```python
from build123d import *

# Parameters (mm, degrees)
SKETCH1_R           = 10
BOSS_EXTRUDE1_DEPTH = 12
SKETCH2_R           = 2
CUT_EXTRUDE1_DEPTH  = 10
SKETCH3_R           = 0.25
BOSS_EXTRUDE2_DEPTH = 10
SKETCH3_3_R         = 0.25
BOSS_EXTRUDE3_DEPTH = 8


with BuildPart() as part:
    # Sketch1 → Boss-Extrude1 (new body)
    with BuildSketch(Plane.XY):
        Circle(SKETCH1_R)
    extrude(amount=BOSS_EXTRUDE1_DEPTH)

    # Sketch2 → Cut-Extrude1 (cut)
    with BuildSketch(Plane.XY.offset(12)):
        Circle(SKETCH2_R)
    extrude(amount=-CUT_EXTRUDE1_DEPTH, mode=Mode.SUBTRACT)

    # Sketch3 → Boss-Extrude2 (add)
    with BuildSketch(Plane(origin=(0, 0, 0), x_dir=(-1, 0, 0), z_dir=(0, 0, -1))):
        with Locations(Location((-8.5, 0, 0), (0, 0, 180))):
            Circle(SKETCH3_R)
    extrude(amount=BOSS_EXTRUDE2_DEPTH)

    # Sketch3_3 → Boss-Extrude3 (add)
    with BuildSketch(Plane(origin=(0, 0, 0), x_dir=(-1, 0, 0), z_dir=(0, 0, -1))):
        with Locations(Location((8.5, 0, 0), (0, 0, 180))):
            Circle(SKETCH3_3_R)
    extrude(amount=BOSS_EXTRUDE3_DEPTH)


solid = part.part
```
Can you work these out from the model? Positions are in its coordinate system, mm. Coordinates: 2 decimals unless noted, no trailing zeros. Order: outer loops, then holes, each group sorted by start corner. A loop starts at its lowest first (then second) coordinate and runs counter-clockwise, first axis right, second up.
1. If we section it at B-B (z = -5.5): Please give me the cut outline in (x, y).
2. I need wall thicknesses on line 1 (Y direction, x = 0, z = 8); line 2 (Y direction, x = -0.75, z = 4); line 3 (Z direction, x = 5.5, y = 7). Which ranges of each line are inside material? Lowest first, please.
3. If we section it at C-C (y = -4): Please give me the cut outline in (x, z), then the cut area to 3 significant figures.
4. If we section it at D-D (x = 3.75): Please give me the cut outline in (y, z), then the cut area to 3 significant figures.
5. Thinking about a two-plate mould opening in X: for faces 1 (the face through (0, -2, 7)), 2 (the face through (-0.1, 2.4, 12)), 3 (the face through (-2.17, -9.76, 5.92)), which applies, +X half, -X half, draft (parallel to the pull), parting line (faces both ways), or undercut?
6. If we section it at A-A (x = 0): Please give me the cut outline in (y, z).
7. I'm going to push flat-ended pins straight in: pin 1 (10 mm diameter, centred on x = -6.5, y = 6.5, fed in from -Z); pin 2 (2 mm diameter, centred on y = 0.5, z = -7, fed in from +X). Where does each tip first touch, or does it pass through?
Entries:
1. outline: circle Ø0.5 at (-8.5, 0); circle Ø0.5 at (8.5, 0)
2. line 1: y = -10 to -2, 2 to 10
2. line 2: y = -9.97 to -1.85, 1.85 to 9.97
2. line 3: z = 0 to 12
3. outline: (-9.17, 0) - (9.17, 0) - (9.17, 12) - (-9.17, 12) - close
3. area: 220 mm2
4. outline: (-9.27, 0) - (9.27, 0) - (9.27, 12) - (-9.27, 12) - close
4. area: 222 mm2
5. face 1: undercut
5. face 2: draft
5. face 3: parting line
6. outline: (-10, 0) - (10, 0) - (10, 12) - (2, 12) - (2, 2) - (-2, 2) - (-2, 12) - (-10, 12) - close
7. pin 1: stops at z = 0
7. pin 2: stops at x = 8.75
